Could you check a few things on this drawing? It's one solid part, dimensions in mm from its lowest x, y, z. Round coordinates to 2 decimals unless told otherwise and drop trailing zeros. Loops run counter-clockwise (first coordinate to the right, second up) from the corner with the lowest first, then second, coordinate; pieces in that order, holes last. Notation, with made-up numbers: M 62,-19.75 L 114,-19.75 A17 ccw 114,-3.75 Z; hole C -10,44.25 d10. An arc over 180 degrees is marked long. Write each question's results on one line, items separated by ' | '. Start each with the question number.
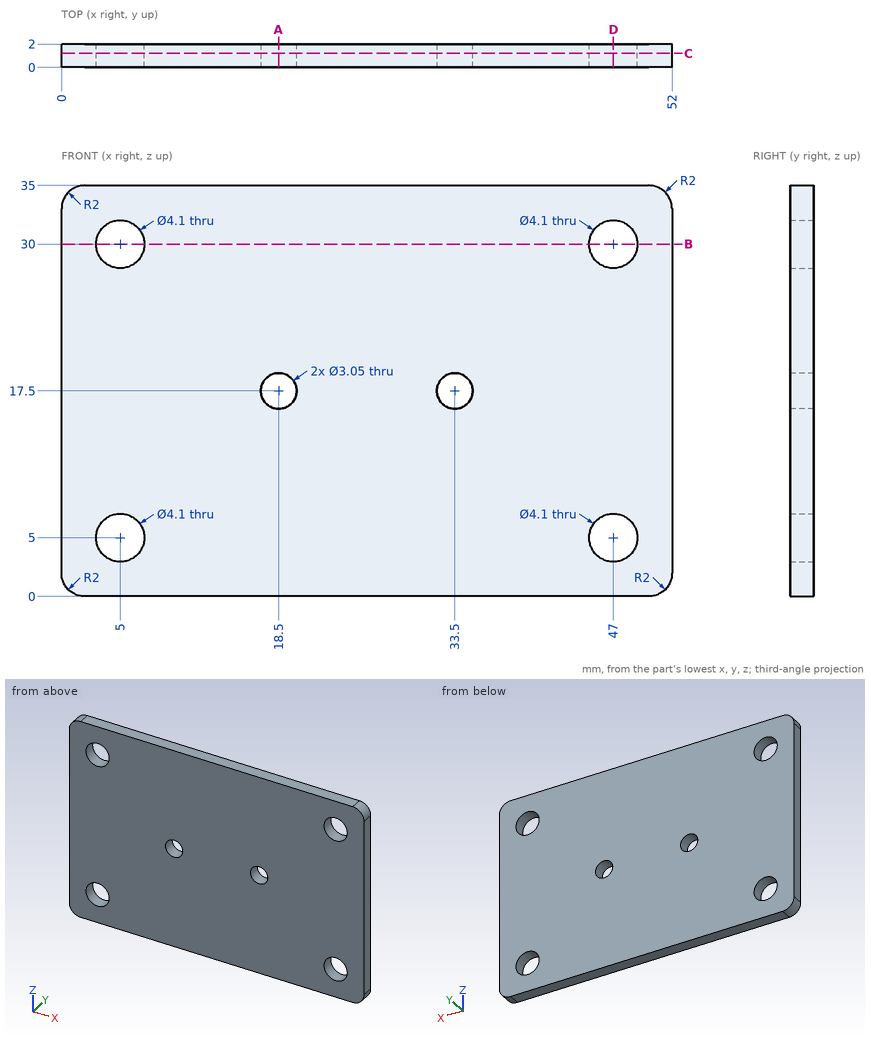
1. I want a section at A-A on x = 18.5. List the corners of the cut face in (y, z) for me (3 decimals).
2. For pin 1 (2.5 mm diameter, centred on x = 33.5, z = 17.5, fed in from -Y), with a flat end and sliding along its axis, tell me the tip position at first contact or that it passes through.
3. I want a section at D-D on x = 47. List the corners of the cut face in (y, z) for me, plus the area to 3 significant figures.
4. I want a section at C-C on y = 1.2. List the corners of the cut face in (x, z) for me (3 decimals).
5. I need wall thicknesses on line 1 along X through (y, z) = (1.1, 17.5) (3 decimals); line 2 along Z through (x, y) = (47, 1.35); line 3 along X through (y, z) = (1.35, 30). Which ranges of each line are inside material? Lowest first, please.
6. I want a section at B-B on z = 30. List the corners of the cut face in (x, y) for me, plus the area to 3 significant figures.
Outcome:
1) outline: M 0,0 L 2,0 L 2,15.975 L 0,15.975 Z; M 0,19.025 L 2,19.025 L 2,35 L 0,35 Z
2) pin 1: through
3) outline: M 0,0 L 2,0 L 2,2.95 L 0,2.95 Z; M 0,7.05 L 2,7.05 L 2,27.95 L 0,27.95 Z; M 0,32.05 L 2,32.05 L 2,35 L 0,35 Z | area: 53.6 mm2
4) outline: M 0,2 A2 ccw 2,0 L 50,0 A2 ccw 52,2 L 52,33 A2 ccw 50,35 L 2,35 A2 ccw 0,33 Z; hole C 5,5 d4.1; hole C 5,30 d4.1; hole C 18.5,17.5 d3.05; hole C 33.5,17.5 d3.05; hole C 47,5 d4.1; hole C 47,30 d4.1
5) line 1: 0 to 16.975, 20.025 to 31.975, 35.025 to 52 | line 2: 0 to 2.95, 7.05 to 27.95, 32.05 to 35 | line 3: 0 to 2.95, 7.05 to 44.95, 49.05 to 52
6) outline: M 0,0 L 2.95,0 L 2.95,2 L 0,2 Z; M 7.05,0 L 44.95,0 L 44.95,2 L 7.05,2 Z; M 49.05,0 L 52,0 L 52,2 L 49.05,2 Z | area: 87.6 mm2
